```python
from build123d import *

# Parameters (mm, degrees)
SKETCH1_R           = 50
BOSS_EXTRUDE1_DEPTH = 10
SKETCH3_R           = 47.5
BOSS_EXTRUDE2_DEPTH = 10
SKETCH5_R           = 2.5
SKETCH6_R           = 2.5
CUT_EXTRUDE1_DEPTH  = 5
CUT_EXTRUDE2_START  = -1
SKETCH7_R           = 47.5
CUT_EXTRUDE2_DEPTH  = 1


with BuildPart() as part:
    # Sketch1 → Boss-Extrude1 (new body)
    with BuildSketch(Plane(origin=(0, 0, 0), x_dir=(1, 0, 0), z_dir=(0, 1, 0))):
        with Locations(Location((0, 0, 0), (0, 0, 270))):
            Circle(SKETCH1_R)
    extrude(amount=BOSS_EXTRUDE1_DEPTH)

    # Sketch3 → Boss-Extrude2 (add)
    with BuildSketch(Plane(origin=(0, 10, 0), x_dir=(1, 0, 0), z_dir=(0, 1, 0))):
        with Locations(Location((0, 0, 0), (0, 0, 270))):
            Circle(SKETCH3_R)
    extrude(amount=BOSS_EXTRUDE2_DEPTH)

    # Cut-Sweep1: sweep along a path in Sketch4
    with BuildLine(Plane(origin=(0, 20, 0), x_dir=(1, 0, 0), z_dir=(0, 1, 0))) as cut_sweep1_path:
        CenterArc((0, 0), 42.5, 0, 360)
    # Sketch5 → Cut-Sweep1 (sweep, cut)
    with BuildSketch(Plane.XY):
        with Locations((42.5, 20)):
            Circle(SKETCH5_R)
    sweep(path=cut_sweep1_path.line, mode=Mode.SUBTRACT)

    # Sketch6 → Cut-Extrude1 (cut)
    with BuildSketch(Plane(origin=(0, 20, 0), x_dir=(1, 0, 0), z_dir=(0, 1, 0))):
        with Locations(Location((0, 0, 0), (0, 0, 270))):
            Circle(SKETCH6_R)
    extrude(amount=-CUT_EXTRUDE1_DEPTH, mode=Mode.SUBTRACT)

    # Sketch7 → Cut-Extrude2 (cut)
    with BuildSketch(Plane(origin=(0, 20, 0), x_dir=(1, 0, 0), z_dir=(0, 1, 0)).offset(CUT_EXTRUDE2_START)):
        with Locations(Location((0, 0, 0), (0, 0, 270))):
            Circle(SKETCH7_R)
    extrude(amount=CUT_EXTRUDE2_DEPTH, mode=Mode.SUBTRACT)


solid = part.part
```
Part model, mm, in its own coordinate system. A direction names the side the tool comes from. Round coordinates to 2 decimals unless told otherwise and drop trailing zeros. Loops run counter-clockwise (first coordinate to the right, second up) from the corner with the lowest first, then second, coordinate; pieces in that order, holes last.
Item 1: 3-axis set-ups, long thin cutter, end or side, ignore diameter. For faces 4 (the face through (-35, 19, -28.4)), 5 (the face through (-18.3, 10, 44.2)): which of +Z, -Z, +X, -X, +Y, -Y reach the whole face in a straight line?
Item 2: Mould opens along X. For faces 1 (the face through (0, 15, 0)), 2 (the face through (-46.37, 14.44, -10.3)), 3 (the face through (1, 0, -1)) say: +X half, -X half, draft (parallel to the pull), parting line (faces both ways), or undercut.
Item 3: Cut at C-C, the plane y = 11.25. Give the cut face in (x, z).
Item 4: Cut at B-B, the plane x = 0. Give the cut face in (y, z), then the cut area to 3 significant figures.
Item 5: Drop flat-ended pins along their axis: P1, Ø5, axis at y = 16, z = 33.5, coming from the +X side; P2, Ø2, axis at y = 5.5, z = 5, coming from the +X side; P3, Ø8, axis at y = 6, z = -6.5, coming from the -X side. Give the stop position or say it passes through.
Item 6: Drill centre lines: line 1 (X direction, y = 17.25, z = 0); line 2 (Y direction, x = 25, z = -42); line 3 (X direction, y = 7, z = -1). Where is each one in solid material? Low to high.
Item 7: Cut at A-A, the plane z = 0. Give the cut face in (x, y).
A:
1. face 4: +Z, -Z, +X, -X, +Y
1. face 5: +Y
2. face 1: undercut
2. face 2: parting line
2. face 3: draft
3. outline: circle Ø95 at (0, 0)
4. outline: (0, -50) - (10, -50) - (10, -47.5) - (19, -47.5) - (19, -44.79) arc R2.5 cw to (19, -40.21) - (19, -2.5) - (15, -2.5) - (15, 2.5) - (19, 2.5) - (19, 40.21) arc R2.5 cw to (19, 44.79) - (19, 47.5) - (10, 47.5) - (10, 50) - (0, 50) - close
4. area: 1,830 mm2
5. P1: stops at x = 35.99
5. P2: stops at x = 49.84
5. P3: stops at x = -49.94
6. line 1: x = -47.5 to -2.5, 2.5 to 47.5
6. line 2: y = 0 to 10
6. line 3: x = -49.99 to 49.99
7. outline: (-50, 0) - (50, 0) - (50, 10) - (47.5, 10) - (47.5, 19) - (44.79, 19) arc R2.5 cw to (40.21, 19) - (2.5, 19) - (2.5, 15) - (-2.5, 15) - (-2.5, 19) - (-40.21, 19) arc R2.5 cw to (-44.79, 19) - (-47.5, 19) - (-47.5, 10) - (-50, 10) - close
